For this review, take the finished solid that the model builds, in its own axes (mm). A direction names the side the tool comes from. Coordinates: 2 decimals unless noted, no trailing zeros. Order: outer loops, then holes, each group sorted by start corner. A loop starts at its lowest first (then second) coordinate and runs counter-clockwise, first axis right, second up. Notation, with made-up numbers: (54.5, -40) -> (61.5, -40) arc R23 cw to (61.5, -6) -> close; hole circle Ø3 at (17, 15). An arc over 180 degrees is marked (long way). Write item = value, one per line. Start each with the question number.
1) Consider section D-D on z = 8.5. Give the boundary of the cut face in (x, y), and give its area (3 significant figures).
2) Consider section A-A on z = 5. Give the boundary of the cut face in (x, y), and give its area (3 significant figures).
3) Insertion check: pin 1 Ø3 at (x, z) = (-2, 6.5) entering from +Y; pin 2 Ø2 at (y, z) = (12.5, 6.5) entering from -X; pin 3 Ø2 at (y, z) = (6.5, 5.5) entering from +X. Each pin has a flat end and moves straight along its axis. Give the tip position at first contact, or say it passes through.
4) Consider section C-C on y = 14. Give the boundary of the cut face in (x, z), and give its area (3 significant figures).
5) Wall thickness on probe 1 along X at (y, z) = (3.25, 5); probe 2 along Z at (x, y) = (14.5, 3); probe 3 along Y at (x, z) = (0.5, 3): over which ranges is each line inside the solid? List them lowest first. Write a range as [from, to].
6) Consider section B-B on x = 0. Give the boundary of the cut face in (y, z).
7) Draft analysis for pull direction Y (two halves, no side actions). For faces 4 (the face through (0, 0, 5)), 5 (the face through (0, 4.181, 5)), 6 (the face through (0, 4, 0)), state which applies: +Y half, -Y half, draft (parallel to the pull), parting line (faces both ways), or undercut.
8) Machinability: for faces 1 (the face through (-13, 5, 4)), 2 (the face through (12.177, 7, 5)), 3 (the face through (0, 17.179, 5)), which of the approach directions +Z, -Z, +X, -X, +Y, -Y give a long, thin tool a straight path to every point of the face, cutting with its end or side? Answer none if there is none.
from build123d import *

# Parameters (mm, degrees)
BOSS_EXTRUDE1_DEPTH = 10
SKETCH2_R           = 2.5
CUT_EXTRUDE1_DEPTH  = 10


with BuildPart() as part:
    # Sketch1 → Boss-Extrude1 (new body)
    with BuildSketch(Plane.XY):
        with BuildLine():
            Line((-16, 0), (16, 0))
            Line((16, 0), (19.18, 0))
            Line((19.18, 0), (19.18, 5))
            Line((19.18, 5), (16, 5))
            Line((16, 5), (12.17699115, 5))
            Line((12.17699115, 5), (12.17699115, 8.995638399))
            ThreePointArc((12.17699115, 8.995638399), (0, 21.172629549), (-12.17699115, 8.995638399))
            Line((-12.17699115, 8.995638399), (-12.17699115, 5))
            Line((-12.17699115, 5), (-16, 5))
            Line((-16, 5), (-19.18, 5))
            Line((-19.18, 5), (-19.18, 0))
            Line((-19.18, 0), (-16, 0))
        make_face()
        Polygon((7.504424779, 10.68), (3.752212389, 17.179022499), (-3.752212389, 17.179022499), (-7.504424779, 10.68), (-3.752212389, 4.180977501), (3.752212389, 4.180977501), align=None, mode=Mode.SUBTRACT)
    extrude(amount=BOSS_EXTRUDE1_DEPTH)

    # Sketch2 → Cut-Extrude1 (cut)
    with BuildSketch(Plane(origin=(0, 5, 0), x_dir=(1, 0, 0), z_dir=(0, 1, 0))):
        with Locations(Location((15.678495575, -5, 0), (0, 0, 270))):
            Circle(SKETCH2_R)
        with Locations(Location((-15.678495575, -5, 0), (0, 0, 270))):
            Circle(SKETCH2_R)
    extrude(amount=-CUT_EXTRUDE1_DEPTH, mode=Mode.SUBTRACT)


solid = part.part
Answer sheet:
q1.outline = (-19.18, 0) -> (19.18, 0) -> (19.18, 5) -> (12.18, 5) -> (12.18, 9) arc R12.18 ccw to (-12.18, 9) -> (-12.18, 5) -> (-19.18, 5) -> close; hole (-7.5, 10.68) -> (-3.75, 4.18) -> (3.75, 4.18) -> (7.5, 10.68) -> (3.75, 17.18) -> (-3.75, 17.18) -> close
q1.area = 376 mm2
q2.outline = (-19.18, 0) -> (-18.18, 0) -> (-18.18, 5) -> (-19.18, 5) -> close; (-13.18, 0) -> (13.18, 0) -> (13.18, 5) -> (12.18, 5) -> (12.18, 9) arc R12.18 ccw to (-12.18, 9) -> (-12.18, 5) -> (-13.18, 5) -> close; (18.18, 0) -> (19.18, 0) -> (19.18, 5) -> (18.18, 5) -> close; hole (-7.5, 10.68) -> (-3.75, 4.18) -> (3.75, 4.18) -> (7.5, 10.68) -> (3.75, 17.18) -> (-3.75, 17.18) -> close
q2.area = 326 mm2
q3.pin_1 = 21.16
q3.pin_2 = -11.92
q3.pin_3 = 12.18
q4.outline = (-11.1, 0) -> (-5.59, 0) -> (-5.59, 10) -> (-11.1, 10) -> close; (5.59, 0) -> (11.1, 0) -> (11.1, 10) -> (5.59, 10) -> close
q4.area = 110 mm2
q5.probe_1 = [-19.18, -18.18], [-13.18, 13.18], [18.18, 19.18]
q5.probe_2 = [0, 2.8], [7.2, 10]
q5.probe_3 = [0, 4.18], [17.18, 21.16]
q6.outline = (0, 0) -> (4.18, 0) -> (4.18, 10) -> (0, 10) -> close; (17.18, 0) -> (21.17, 0) -> (21.17, 10) -> (17.18, 10) -> close
q7.face_4 = -Y half
q7.face_5 = undercut
q7.face_6 = draft
q8.face_1 = +Z, -Z, -X, +Y
q8.face_2 = +Z, -Z, +X, +Y
q8.face_3 = +Z, -Z
